Part model, mm, in its own coordinate system. A direction names the side the tool comes from. Coordinates: 2 decimals unless noted, no trailing zeros. Write each loop counter-clockwise with the first axis right and the second up, starting at its lowest first coordinate (ties: lowest second). Pieces come first, ordered by that corner, then holes. Notation, with made-up numbers: M 40.25,-22.5 L 44.25,-22.5 A20 cw 44.25,-0.5 Z; hole C -9.5,14 d9. An arc over 180 degrees is marked long. Use a Markdown table: item, result. Add a question column.
Q1. Pin check, flat tips, straight feed: pin 1 Ø1.2 at (x, z) = (4.5, 2) entering from +Y; pin 2 Ø0.9 at (x, z) = (3, 2.5) entering from +Y; pin 3 Ø1 at (x, z) = (15.5, 1.5) entering from -Y. Stop position of each tip, or through.
Q2. Wall check: L1, parallel to X at y = 3.5, z = 1.25; L2, parallel to Y at x = 12, z = 2.35; L3, parallel to Y at x = 11, z = 0.3. Give the ranges that are in metal, low to high. Write a range as from..to.
Q3. Mould opens along X. For faces 3 (the flat face through (7.5, 10, 2)), 4 (the flat face through (1.48, 10, 2)), 5 (the cylindrical face through (16.8, 15.94, 1.97)), 6 (the flat face through (13, 8.991, 2)) say: released by +X, released by -X, zero draft, split by the parting line, or undercut.
Q4. Slice it at A-A on y = 10.5. Write the cut outline in (x, z), then the cut area to 3 significant figures.
Q5. Slice it at C-C on z = 1.2. Write the cut outline in (x, y).
Q6. Slice it at B-B on y = 3. Write the cut outline in (x, z), then the cut area to 3 significant figures.
Q7. Slice it at D-D on x = 15. Write the cut outline in (y, z), then the cut area to 3 significant figures.
Q8. Tool access for faces 1 (the flat face through (6.94, 13.71, 1.97)), 2 (the cylindrical face through (9.044, 0.012, 1.972)): list every direction of +Z, -Z, +X, -X, +Y, -Y with a clear straight run to the whole face (end or side of a thin tool).
from build123d import *

# Parameters (mm, degrees)
SKETCH1_W           = 4
SKETCH1_H           = 2
BOSS_EXTRUDE1_DEPTH = 4


with BuildPart() as part:
    # Sketch1 → Boss-Extrude1 (new body)
    with BuildSketch(Plane.XY):
        with BuildLine():
            Line((14.475572066, 6), (15.475572066, 7.732050808))
            Line((15.475572066, 7.732050808), (17.939673681, 6.309401077))
            Line((17.939673681, 6.309401077), (17.939673681, 13.142551265))
            ThreePointArc((17.939673681, 13.142551265), (16.768100806, 15.97097839), (13.939673681, 17.142551265))
            ThreePointArc((13.939673681, 17.142551265), (9.2, 20.197069168), (4.460326319, 17.142551265))
            Line((4.460326319, 17.142551265), (1.48, 17.142551265))
            Line((1.48, 17.142551265), (1.48, 2))
            ThreePointArc((1.48, 2), (9.155654032, 0.008565204), (16.939673681, 1.522010102))
            Line((16.939673681, 1.522010102), (16.939673681, 4.577350269))
            Line((16.939673681, 4.577350269), (14.475572066, 6))
        make_face()
        with Locations((5.5, 9.99107808)):
            Rectangle(SKETCH1_W, SKETCH1_H, mode=Mode.SUBTRACT)
        with Locations((9.111056117, 3.09107808)):
            Rectangle(SKETCH1_W, SKETCH1_H, mode=Mode.SUBTRACT)
        with Locations((13.5, 9.99107808)):
            Rectangle(SKETCH1_W, SKETCH1_H, mode=Mode.SUBTRACT)
        Polygon((6.2, 14.99107808), (7.7, 12.393001869), (10.7, 12.393001869), (12.2, 14.99107808), (10.7, 17.589154291), (7.7, 17.589154291), align=None, mode=Mode.SUBTRACT)
    extrude(amount=BOSS_EXTRUDE1_DEPTH)


solid = part.part
Recorded:
| question | item | result |
|---|---|---|
| 1 | pin 1 | y = 18.2 |
| 1 | pin 2 | y = 17.14 |
| 1 | pin 3 | y = 0.8 |
| 2 | L1 | 1.48..7.11, 11.11..16.94 |
| 2 | L2 | 0.15..8.99, 10.99..14.64, 15.34..19.38 |
| 2 | L3 | 0.05..2.09, 4.09..12.91, 17.07..19.88 |
| 3 | face 3 | undercut |
| 3 | face 4 | released by -X |
| 3 | face 5 | released by +X |
| 3 | face 6 | undercut |
| 4 | outline | M 1.48,0 L 3.5,0 L 3.5,4 L 1.48,4 Z; M 7.5,0 L 11.5,0 L 11.5,4 L 7.5,4 Z; M 15.5,0 L 17.94,0 L 17.94,4 L 15.5,4 Z |
| 4 | area | 33.8 mm² |
| 5 | outline | M 1.48,2 A17.93 ccw 16.94,1.52 L 16.94,4.58 L 14.48,6 L 15.48,7.73 L 17.94,6.31 L 17.94,13.14 A4 ccw 13.94,17.14 A5.2 ccw 4.46,17.14 L 1.48,17.14 Z; hole M 3.5,8.99 L 7.5,8.99 L 7.5,10.99 L 3.5,10.99 Z; hole M 6.2,14.99 L 7.7,12.39 L 10.7,12.39 L 12.2,14.99 L 10.7,17.59 L 7.7,17.59 Z; hole M 7.11,2.09 L 11.11,2.09 L 11.11,4.09 L 7.11,4.09 Z; hole M 11.5,8.99 L 15.5,8.99 L 15.5,10.99 L 11.5,10.99 Z |
| 6 | outline | M 1.48,0 L 7.11,0 L 7.11,4 L 1.48,4 Z; M 11.11,0 L 16.94,0 L 16.94,4 L 11.11,4 Z |
| 6 | area | 45.8 mm² |
| 7 | outline | M 0.8,0 L 5.7,0 L 5.7,4 L 0.8,4 Z; M 6.91,0 L 8.99,0 L 8.99,4 L 6.91,4 Z; M 10.99,0 L 17,0 L 17,4 L 10.99,4 Z |
| 7 | area | 52.0 mm² |
| 8 | face 1 | +Z, -Z |
| 8 | face 2 | +Z, -Z, -Y |
